For this review, use the dimensioned drawing (mm, ordinates from the lowest corner) and the shaded views. A direction names the side the tool comes from. Round coordinates to 2 decimals unless told otherwise and drop trailing zeros. Loops run counter-clockwise (first coordinate to the right, second up) from the corner with the lowest first, then second, coordinate; pieces in that order, holes last. Notation, with made-up numbers: M -29,79 L -8,79 A15 ccw -8,92 Z; hole C -1,82 d2. An arc over 180 degrees is marked long. Write item = value, one per line. Start each with the question number.
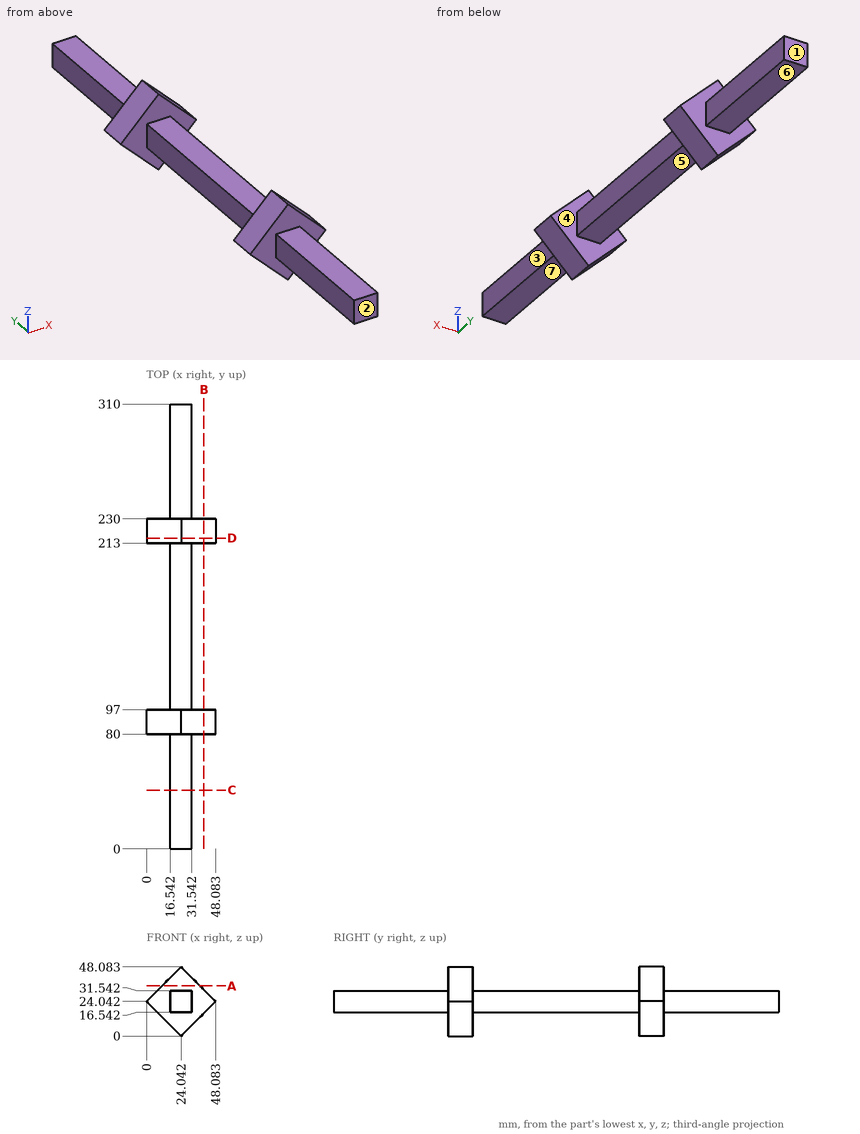
(1) Add section C-C on y = 41. Write out the cut boundary in (x, z).
(2) Add section A-A on z = 35. Write out the cut boundary in (x, y) (1 decimal), and give its area (3 significant figures).
(3) Draft analysis for pull direction Y (two halves, no side actions). For the marked faces 1, 2, 3 and 4, state which applies: +Y half, -Y half, draft (parallel to the pull), parting line (faces both ways), or undercut.
(4) Add section D-D on y = 216.5. Write out the cut boundary in (x, z), and give its area (3 significant figures).
(5) Wall thickness on L1, parallel to Y at x = 9.5, z = 28; L2, parallel to Z at x = 25, y = 134.5: over which ranges is each line inside the solid? List them lowest first.
(6) Add section B-B on x = 40. Write out the cut boundary in (y, z) (1 decimal), and give its area (3 significant figures).
(7) Tool access review of the marked faces 5, 6 and 7: name each direction out of +Z, -Z, +X, -X, +Y, -Y from which nothing blocks a thin tool from reaching the whole face with its end or side.
(8) For pin 1 Ø12 at (y, z) = (251.5, 26) entering from +X; pin 2 Ø1.5 at (x, z) = (8.5, 15) entering from +Y; pin 3 Ø7.5 at (y, z) = (166, 25.5) entering from -X, all flat-tipped, find the tip position at first contact; note any pin that passes through.
Answer sheet:
q1.outline = M 16.54,16.54 L 31.54,16.54 L 31.54,31.54 L 16.54,31.54 Z
q2.outline = M 11,80 L 37.1,80 L 37.1,97 L 11,97 Z; M 11,213 L 37.1,213 L 37.1,230 L 11,230 Z
q2.area = 890 mm²
q3.face_1 = +Y half
q3.face_2 = -Y half
q3.face_3 = draft
q3.face_4 = undercut
q4.outline = M 0,24.04 L 24.04,0 L 48.08,24.04 L 24.04,48.08 Z
q4.area = 1,160 mm²
q5.L1 = 80 to 97, 213 to 230
q5.L2 = 16.54 to 31.54
q6.outline = M 80,16 L 97,16 L 97,32.1 L 80,32.1 Z; M 213,16 L 230,16 L 230,32.1 L 213,32.1 Z
q6.area = 550 mm²
q7.face_5 = -Z, +X, -X
q7.face_6 = -Z, +X, -X, +Y
q7.face_7 = -Z, +X, -X, -Y
q8.pin_1 = 31.54
q8.pin_2 = 230
q8.pin_3 = 16.54
